Part model, mm, in its own coordinate system. Round coordinates to 2 decimals unless told otherwise and drop trailing zeros. Loops run counter-clockwise (first coordinate to the right, second up) from the corner with the lowest first, then second, coordinate; pieces in that order, holes last. Notation, with made-up numbers: (10.5, -30) -> (32.5, -30) arc R34 ccw to (32.5, 4) -> close; hole circle Ø7 at (50.5, -28). An arc over 180 degrees is marked (long way). Use a Markdown table: item, result. Add a question column.
Item 1: Cut at D-D, the plane x = 8.5. List the corners of the cut face in (y, z).
Item 2: Two-plate mould, pull along Z, no slides. Class faces 1 (the face through (14.06, 12.67, -24.37)), 2 (the face through (-1, -28.3, 11.9)), 3 (the face through (10.01, 31, 9.76)): pulls with the +Z half, pulls with the -Z half, needs draft (parallel to the pull), parting line crosses it, or undercut.
Item 3: Probe line 1 (Y direction, x = 18, z = -10); line 2 (Z direction, x = 6, y = 18); line 3 (Y direction, x = 8, z = 18.5). List the from-to ranges inside material, lowest first. Write a range as [from, to].
Item 4: Cut at C-C, the plane x = 14.25. List the corners of the cut face in (y, z).
Item 5: Cut at A-A, the plane z = 0. List the corners of the cut face in (x, y).
Item 6: Flat gauge pins, fed straight in: pin 1 (10 mm diameter, centred on x = 10, z = 21.5, fed in from -Y); pin 2 (3 mm diameter, centred on x = 19, y = 25.5, fed in from -Z); pin 3 (4 mm diameter, centred on x = 17.5, z = 5, fed in from -Y). Where does each tip first touch, or does it go through?
```python
from build123d import *

# Parameters (mm, degrees)
FILLET1_R = 1.5
FILLET2_R = 0.8
FILLET3_R = 0.4


with BuildPart() as part:
    # Sketch1 → Revolve1 (revolve)
    with BuildSketch(Plane.XY):
        Polygon((22, 26.5), (22, 32.5), (-1, 32.5), (-1, 30.120326542), (19.5318921, 26.5), align=None)
    revolve(axis=Axis((0, 0, 0), (1, 0, 0)))

    # Fillet1
    fillet1_edges = [part.edges().sort_by_distance(p)[0] for p in [
        (22, -32.5, 0),
    ]]
    fillet(fillet1_edges, radius=FILLET1_R)

    # Fillet2
    fillet2_edges = [part.edges().sort_by_distance(p)[0] for p in [
        (-1, -32.5, 0),
    ]]
    fillet(fillet2_edges, radius=FILLET2_R)

    # Fillet3
    fillet3_edges = [part.edges().sort_by_distance(p)[0] for p in [
        (22, -26.5, 0),
        (-1, -30.120326542, 0),
    ]]
    fillet(fillet3_edges, radius=FILLET3_R)


solid = part.part
```
A:
| question | item | result |
|---|---|---|
| 1 | outline | circle Ø65 at (0, 0); hole circle Ø56.89 at (0, 0) |
| 2 | face 1 | undercut |
| 2 | face 2 | needs draft |
| 2 | face 3 | parting line crosses it |
| 3 | line 1 | y = [-30.92, -24.83], [24.83, 30.92] |
| 3 | line 2 | z = [-27.06, -22.59], [22.59, 27.06] |
| 3 | line 3 | y = [-26.72, -21.72], [21.72, 26.72] |
| 4 | outline | circle Ø65 at (0, 0); hole circle Ø54.86 at (0, 0) |
| 5 | outline | (-1, -31.7) arc R0.8 ccw to (-0.2, -32.5) -> (20.5, -32.5) arc R1.5 ccw to (22, -31) -> (22, -26.9) arc R0.4 ccw to (21.6, -26.5) -> (19.53, -26.5) -> (-0.67, -30.06) arc R0.4 ccw to (-1, -30.46) -> close; (-1, 30.46) arc R0.4 ccw to (-0.67, 30.06) -> (19.53, 26.5) -> (21.6, 26.5) arc R0.4 ccw to (22, 26.9) -> (22, 31) arc R1.5 ccw to (20.5, 32.5) -> (-0.2, 32.5) arc R0.8 ccw to (-1, 31.7) -> close |
| 6 | pin 1 | stops at y = -28 |
| 6 | pin 2 | stops at z = -21.91 |
| 6 | pin 3 | stops at y = -32.36 |
